from build123d import *

# Parameters (mm, degrees)
F0_W     = 71
F0_H     = 54
F1_DEPTH = 97
F2_T     = -2
F4_DEPTH = 97
F6_DEPTH = 71
F7_R     = 1.19999


# Not quite as in the source:
# - a fillet or chamfer is up to 0.001 mm smaller than in the source, because OpenCascade refuses the exact size


with BuildPart() as f1:
    # F0 (on Front) → F1 (new body)
    with BuildSketch(Plane.XZ):
        with Locations((35.5, -27)):
            Rectangle(F0_W, F0_H)
    extrude(amount=-F1_DEPTH)

    # F2
    f2_openings = [f1.faces().sort_by_distance(p)[0] for p in [
        (35.5, 48.5, 0),
    ]]
    offset(amount=F2_T, openings=f2_openings)

    # F3 (on face) → F4 (join, through all)
    with BuildSketch(Plane.XZ):
        Polygon((0, 2), (0, 0), (1.2, 0), (2, 1), (2, 2), align=None)
        Polygon((69, 1), (69.8, 0), (71, 0), (71, 2), (69, 2), align=None)
    extrude(amount=-F4_DEPTH)

    # F5 (on face) → F6 (join, through all)
    with BuildSketch(Plane.YZ.offset(71)):
        Polygon((97, 0), (97, 2), (95, 2), (95, 1), (95.8, 0), align=None)
    extrude(amount=-F6_DEPTH)

    # F7 (radius 1.2 in the source; OpenCascade refuses exactly that, so slightly less here)
    f7_edges = [f1.edges().sort_by_distance(p)[0] for p in [
        (71, 0, -26),
        (71, 97, -26),
        (0, 0, -26),
        (0, 97, -26),
    ]]
    fillet(f7_edges, radius=F7_R)


solid = f1.part
Could you check a few things on this model? Use its own coordinates, in mm. A direction names the side the tool comes from. Give positions to 0.01 mm unless a question says otherwise; leave off trailing zeros. Write each loop counter-clockwise with the first axis right and the second up, starting at its lowest first coordinate (ties: lowest second). Pieces come first, ordered by that corner, then holes. Notation, with made-up numbers: (60, 21.5) -> (115, 21.5) arc R6 ccw to (115, 27.5) -> close; hole circle Ø9 at (0, 85). An arc over 180 degrees is marked (long way). Answer as CSV lines item,"result". Start each with the question number.
(1) If we section it at B-B, the plane y = 56: Write out the boundary of the cut face in (x, z), and give its area (3 significant figures).
(2) Please list where these lines run through material, in increasing order: line 1 (Y direction, x = 29, z = -50); line 2 (X direction, y = 32.5, z = -29.5); line 3 (Z direction, x = 17.5, y = 44.5).
(3) If we section it at A-A, the plane z = -40.5: Write out the boundary of the cut face in (x, y).
(4) If we section it at C-C, the plane x = 50.5: Write out the boundary of the cut face in (y, z), and give its area (3 significant figures).
(5) If we mould it in two halves opening along X, with no side actions, what happens to faces 3 (the face through (71, 48, -26)), 4 (the face through (0, 48, -26)), 5 (the face through (2, 48, -26))? For each: +X half, -X half, draft (parallel to the pull), parting line (faces both ways), or undercut.
(6) I'm going to push a flat-ended pin straight in: pin 1 Ø0.8 at (x, z) = (41.5, 1.5) entering from -Y. Where does the tip first touch, or does it pass through?
(7) Which directions (+Z, -Z, +X, -X, +Y, -Y) give clear straight access to the entire face, cutting with the end or side of a thin tool? Please do faces 1 (the face through (35, 48, -54)), 2 (the face through (69, 48, -26)).
Answer list:
1,outline,"(0, -54) -> (71, -54) -> (71, 2) -> (69, 2) -> (69, 1) -> (69.8, 0) -> (69, 0) -> (69, -52) -> (2, -52) -> (2, 0) -> (1.2, 0) -> (2, 1) -> (2, 2) -> (0, 2) -> close"
1,area,"357 mm^2"
2,line 1,"0 to 2, 95 to 97"
2,line 2,"0 to 2, 69 to 71"
2,line 3,"-54 to -52"
3,outline,"(0, 1.2) arc R1.2 ccw to (1.2, 0) -> (69.8, 0) arc R1.2 ccw to (71, 1.2) -> (71, 95.8) arc R1.2 ccw to (69.8, 97) -> (1.2, 97) arc R1.2 ccw to (0, 95.8) -> close; hole (2, 2) -> (69, 2) -> (69, 95) -> (2, 95) -> close"
4,outline,"(0, -54) -> (97, -54) -> (97, 2) -> (95, 2) -> (95, 1) -> (95.8, 0) -> (95, 0) -> (95, -52) -> (2, -52) -> (2, 0) -> (0, 0) -> close"
4,area,"406 mm^2"
5,face 3,"+X half"
5,face 4,"-X half"
5,face 5,"undercut"
6,pin 1,"y = 95"
7,face 1,"-Z, +X, -X, +Y, -Y"
7,face 2,"+Z"
